Design review of the part built by this model. Coordinates are the model's own, in mm. Face numbers are marked on the shaded views. A direction names the side the tool comes from. Coordinates: 2 decimals unless noted, no trailing zeros. Order: outer loops, then holes, each group sorted by start corner. A loop starts at its lowest first (then second) coordinate and runs counter-clockwise, first axis right, second up. Notation, with made-up numbers: M -9,75 L 21,75 A31 cw 21,108 Z; hole C -2,52 d7. An arc over 180 degrees is marked long. Answer in a Markdown table with one row per item.
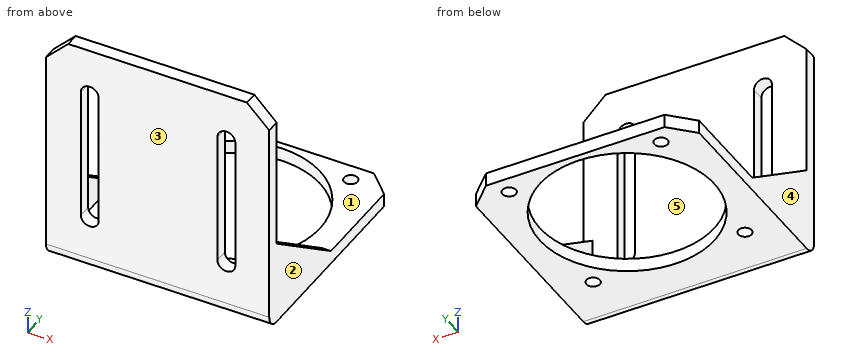
from build123d import *

# Parameters (mm, degrees)
SKETCH_1_R      = 1.5
SKETCH_1_R_2    = 19.5
EXTRUDE_1_DEPTH = 3
EXTRUDE_3_DEPTH = 3
EXTRUDE_4_DEPTH = 2
FILLET_2_R      = 3


with BuildPart() as part:
    # 草图1 → 凸台-拉伸1 (new body)
    with BuildSketch(Plane.XY):
        Polygon((20, 25.75), (-20, 25.75), (-25, 20.75), (-25, -25.75), (25, -25.75), (25, 20.75), align=None)
        with Locations((-17, -12.25)):
            Circle(SKETCH_1_R, mode=Mode.SUBTRACT)
        with Locations((17, -12.25)):
            Circle(SKETCH_1_R, mode=Mode.SUBTRACT)
        with Locations((-17, 21.75)):
            Circle(SKETCH_1_R, mode=Mode.SUBTRACT)
        with Locations((0, 4.75)):
            Circle(SKETCH_1_R_2, mode=Mode.SUBTRACT)
        with Locations((17, 21.75)):
            Circle(SKETCH_1_R, mode=Mode.SUBTRACT)
    extrude(amount=EXTRUDE_1_DEPTH)

    # 草图2 → 凸台-拉伸3 (add)
    with BuildSketch(Plane.XZ.offset(25.75)):
        Polygon((-25, 48.5), (-25, 0), (25, 0), (25, 48.5), (20, 53.5), (-20, 53.5), align=None)
        with BuildLine():
            ThreePointArc((-13.2, 12.8), (-15.2, 10.8), (-17.2, 12.8))
            Line((-17.2, 12.8), (-17.2, 42.8))
            ThreePointArc((-17.2, 42.8), (-15.2, 44.8), (-13.2, 42.8))
            Line((-13.2, 42.8), (-13.2, 12.8))
        make_face(mode=Mode.SUBTRACT)
        with BuildLine():
            ThreePointArc((17.4, 12.8), (15.4, 10.8), (13.4, 12.8))
            Line((13.4, 12.8), (13.4, 42.8))
            ThreePointArc((13.4, 42.8), (15.4, 44.8), (17.4, 42.8))
            Line((17.4, 42.8), (17.4, 12.8))
        make_face(mode=Mode.SUBTRACT)
    extrude(amount=-EXTRUDE_3_DEPTH)

    # 草图3 → 凸台-拉伸4 (add)
    with BuildSketch(Plane(origin=(25, 0, 0), x_dir=(0, 0, -1), z_dir=(1, 0, 0))):
        Polygon((-3, -0.75), (-3, -22.75), (-19, -22.75), align=None)
    extrude_4 = extrude(amount=-EXTRUDE_4_DEPTH)

    # 镜向1: 凸台-拉伸4 across plane
    add(extrude_4.mirror(Plane(origin=(0, 0, 0), x_dir=(0, 0, 1), z_dir=(1, 0, 0))))

    # 圆角2
    fillet_2_edges = [part.edges().sort_by_distance(p)[0] for p in [
        (0, -25.75, 0),
        (0, -22.75, 3),
    ]]
    fillet(fillet_2_edges, radius=FILLET_2_R)


solid = part.part
(1) Add section A-A, the plane y = 4.75. Give the boundary of the cut face in (x, z).
Return value:
| item | result |
|---|---|
| outline | M -25,0 L -19.5,0 L -19.5,3 L -25,3 Z; M 19.5,0 L 25,0 L 25,3 L 19.5,3 Z |
(2) Add section C-C, the plane z = 44. Give the boundary of the cut face in (x, y).
Return value:
| item | result |
|---|---|
| outline | M -25,-25.75 L -16.8,-25.75 L -16.8,-22.75 L -25,-22.75 Z; M -13.6,-25.75 L 13.8,-25.75 L 13.8,-22.75 L -13.6,-22.75 Z; M 17,-25.75 L 25,-25.75 L 25,-22.75 L 17,-22.75 Z |
(3) For line 1 along X through (y, z) = (-23.5, 13); line 2 along X through (y, z) = (-12, 1); line 3 along X through (y, z) = (-21, 5.5), list the stretches that pass through material, from the lowest coordinate up. Write a range as from..to.
Return value:
| item | result |
|---|---|
| line 1 | x = -25..-17.2, -13.2..13.4, 17.4..25 |
| line 2 | x = -25..-18.48, -15.52..-9.98, 9.98..15.52, 18.48..25 |
| line 3 | x = -25..-23, 23..25 |
(4) Draft analysis for pull direction X (two halves, no side actions). For the marked faces 3, 4 and 5, state which applies: pulls with the +X half, pulls with the -X half, needs draft (parallel to the pull), parting line crosses it, or undercut.
Return value:
| item | result |
|---|---|
| face 3 | needs draft |
| face 4 | pulls with the -X half |
| face 5 | undercut |
(5) For the marked faces 1 and 2, list the 3-axis set-ups (+Z, -Z, +X, -X, +Y, -Y) from which the entire face can be reached by the end or side of a thin tool; tool diameter is ignored.
Return value:
| item | result |
|---|---|
| face 1 | +Z, +Y |
| face 2 | +Z, -Z, +X, +Y, -Y |
(6) Add section B-B, the plane x = 0. Give the boundary of the cut face in (y, z).
Return value:
| item | result |
|---|---|
| outline | M -25.75,3 A3 ccw -22.75,0 L -14.75,0 L -14.75,3 L -19.75,3 A3 cw -22.75,6 L -22.75,53.5 L -25.75,53.5 Z; M 24.25,0 L 25.75,0 L 25.75,3 L 24.25,3 Z |
(7) Add section D-D, the plane y = 21.75. Give the boundary of the cut face in (x, z), and give its area (3 significant figures).
Return value:
| item | result |
|---|---|
| outline | M -24,0 L -18.5,0 L -18.5,3 L -24,3 Z; M -15.5,0 L -9.55,0 L -9.55,3 L -15.5,3 Z; M 9.55,0 L 15.5,0 L 15.5,3 L 9.55,3 Z; M 18.5,0 L 24,0 L 24,3 L 18.5,3 Z |
| area | 68.7 mm2 |
(8) Insertion check: pin 1 Ø3 at (x, y) = (15.5, 17) entering from +Z; pin 2 Ø3.5 at (x, y) = (-17, 21.75) entering from -Z; pin 3 Ø1 at (x, z) = (-13.5, 20) entering from +Y. Each pin has a flat end and moves straight along its axis. Give the tip position at first contact, or say it passes through.
Return value:
| item | result |
|---|---|
| pin 1 | stops at z = 3 |
| pin 2 | stops at z = 0 |
| pin 3 | stops at y = -22.75 |
